from build123d import *

# Parameters (mm, degrees)
BOSS_EXTRUDE1_DEPTH = 133.35
FILLET1_R           = 31.75
SHELL1_T            = -3.175


with BuildPart() as part:
    # Sketch1 → Boss-Extrude1 (new body)
    with BuildSketch(Plane(origin=(0, 0, 0), x_dir=(1, 0, 0), z_dir=(0, 1, 0))):
        Polygon((0, 0), (0, 155.575), (-82.55, 155.575), (-82.55, -82.55), (155.575, -82.55), (155.575, 0), align=None)
    extrude(amount=BOSS_EXTRUDE1_DEPTH)

    # Fillet1
    fillet1_edges = [part.edges().sort_by_distance(p)[0] for p in [
        (-82.55, 66.675, 82.55),
        (-82.55, 133.35, -36.5125),
        (36.5125, 133.35, 82.55),
        (36.5125, 0, 82.55),
        (-82.55, 0, -36.5125),
    ]]
    fillet(fillet1_edges, radius=FILLET1_R)

    # Shell1
    shell1_openings = [part.faces().sort_by_distance(p)[0] for p in [
        (0, 66.675, -77.7875),
        (77.7875, 66.675, 0),
    ]]
    offset(amount=SHELL1_T, openings=shell1_openings, kind=Kind.INTERSECTION)


solid = part.part
Read the model definition and answer for the solid it produces. Units are mm, in the model's axes. A direction names the side the tool comes from. Round coordinates to 2 decimals unless told otherwise and drop trailing zeros. Order: outer loops, then holes, each group sorted by start corner. A loop starts at its lowest first (then second) coordinate and runs counter-clockwise, first axis right, second up.
1) The part is cut by section C-C on y = 87. Write down the section's boundary in (x, z) (3 decimals).
2) The mould has two halves that part along Y. Classify faces 1 (the face through (5, 0, 15)), 2 (the face through (49, 66, 79.375)), 3 (the face through (0, 2, -77)): released by +Y, released by -Y, zero draft, split by the parting line, or undercut.
3) The part is cut by section A-A on x = -41.5. Write down the section's boundary in (y, z) (3 decimals), plus the area to 3 significant figures.
4) For faces 4 (the face through (52.22, 11.77, 71.23)), 5 (the face through (-39, 66, -152.4)), 6 (the face through (-73.5, 67.2, 73)), determine the directions among +Z, -Z, +X, -X, +Y, -Y from which every point of the face is accessible in a straight line to the end or side of a thin tool.
5) Straight lines are drawn through the part: L1, parallel to X at y = 83, z = 1 (3 decimals); L2, parallel to Y at x = 51, z = 32 (3 decimals); L3, parallel to Z at x = -35.5, y = 53.5 (3 decimals). For each, find the intervals that lie inside material, in ascending order.
6) The part is cut by section B-B on z = 25.5. Write down the section's boundary in (x, y) (3 decimals), plus the area to 3 significant figures.
7) Flat-ended cylindrical pins translate along their axes: pin 1 (8 mm diameter, centred on y = 80, z = -107.5, fed in from +X) (3 decimals); pin 2 (6 mm diameter, centred on x = 83.5, y = 70.5, fed in from -Z) (3 decimals); pin 3 (5 mm diameter, centred on y = 21, z = -96.5, fed in from +X). Find the tip coordinate at first contact, or state that the pin passes through.
8) The part is cut by section D-D on x = 125. Write down the section's boundary in (y, z) (3 decimals).
Resolved:
1. outline: (-82.55, -155.575) - (0, -155.575) - (0, -152.4) - (-79.375, -152.4) - (-79.375, 50.8) arc R28.575 cw to (-50.8, 79.375) - (152.4, 79.375) - (152.4, 0) - (155.575, 0) - (155.575, 82.55) - (-50.8, 82.55) arc R31.75 ccw to (-82.55, 50.8) - close
2. face 1: released by -Y
2. face 2: undercut
2. face 3: zero draft
3. outline: (0, -155.575) - (133.35, -155.575) - (133.35, 50.8) arc R31.75 ccw to (101.6, 82.55) - (31.75, 82.55) arc R31.75 ccw to (0, 50.8) - close; hole (3.175, -152.4) - (130.175, -152.4) - (130.175, 50.8) arc R28.575 ccw to (101.6, 79.375) - (31.75, 79.375) arc R28.575 ccw to (3.175, 50.8) - close
3. area: 2,240 mm2
4. face 4: none
4. face 5: +X
4. face 6: +Z, -X, +Y, -Y
5. L1: x = -82.55 to -79.375, 152.4 to 155.575
5. L2: y = 0 to 3.175, 130.175 to 133.35
5. L3: z = -155.575 to -152.4, 79.375 to 82.55
6. outline: (-82.55, 31.75) arc R31.75 ccw to (-50.8, 0) - (155.575, 0) - (155.575, 133.35) - (-50.8, 133.35) arc R31.75 ccw to (-82.55, 101.6) - close; hole (-79.375, 31.75) arc R28.575 ccw to (-50.8, 3.175) - (152.4, 3.175) - (152.4, 130.175) - (-50.8, 130.175) arc R28.575 ccw to (-79.375, 101.6) - close
6. area: 2,240 mm2
7. pin 1: stops at x = -79.375
7. pin 2: stops at z = 79.375
7. pin 3: stops at x = -76.12
8. outline: (0, 0) - (3.175, 0) - (3.175, 50.8) arc R28.575 cw to (31.75, 79.375) - (101.6, 79.375) arc R28.575 cw to (130.175, 50.8) - (130.175, 0) - (133.35, 0) - (133.35, 50.8) arc R31.75 ccw to (101.6, 82.55) - (31.75, 82.55) arc R31.75 ccw to (0, 50.8) - close
